```python
from build123d import *

# Parameters (mm, degrees)
SKETCH3_W                                    = 60
SKETCH3_H                                    = 30
BOSS_EXTRUDE1_DEPTH                          = 10
CBORE_FOR_M6_HEX_HEAD_CAP_SCREW1_D           = 6.6
CBORE_FOR_M6_HEX_HEAD_CAP_SCREW1_CBORE_D     = 10.5
CBORE_FOR_M6_HEX_HEAD_CAP_SCREW1_CBORE_DEPTH = 7.5
CUT_EXTRUDE1_DEPTH                           = 10


with BuildPart() as part:
    # Sketch3 → Boss-Extrude1 (new, symmetric)
    with BuildSketch(Plane.XY):
        Rectangle(SKETCH3_W, SKETCH3_H)
    extrude(amount=BOSS_EXTRUDE1_DEPTH, both=True)

    # CBORE for M6 Hex Head Cap Screw1 (through all)
    with Locations(Plane(origin=(0, 0, -10), x_dir=(-1, 0, 0), z_dir=(0, 0, -1))):
        with Locations((18, 0), (-18, 0)):
            CounterBoreHole(CBORE_FOR_M6_HEX_HEAD_CAP_SCREW1_D / 2, CBORE_FOR_M6_HEX_HEAD_CAP_SCREW1_CBORE_D / 2, CBORE_FOR_M6_HEX_HEAD_CAP_SCREW1_CBORE_DEPTH)

    # Sketch9 → Tap Drill for M12 Tap1 (revolve, cut)
    with BuildSketch(Plane(origin=(0, 0, -10), x_dir=(0, 1, 0), z_dir=(1, 0, 0))):
        Polygon((0, 0), (0, 20), (5.125, 20), (5.1, 19.975), (5.1, 0.025), (5.125, 0), align=None)
    revolve(axis=Axis((0, 0, -16.35), (0, 0, 1)), mode=Mode.SUBTRACT)

    # Sketch11 → Cut-Extrude1 (cut)
    with BuildSketch(Plane(origin=(0, 0, 10), x_dir=(-1, 0, 0), z_dir=(0, 0, -1))):
        Polygon((4.907477288, 8.5), (-4.907477288, 8.5), (-9.814954576, 0), (-4.907477288, -8.5), (4.907477288, -8.5), (9.814954576, 0), align=None)
    extrude(amount=CUT_EXTRUDE1_DEPTH, mode=Mode.SUBTRACT)


solid = part.part
```
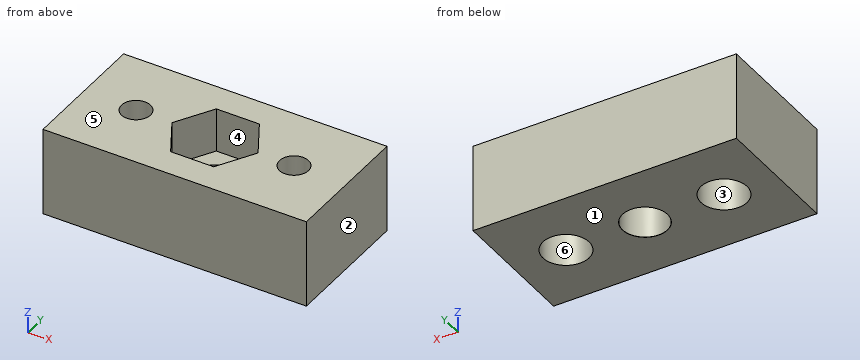
Input: part model. Units: mm. Frame: model coordinates. Face numbers are marked on the shaded views. A direction names the side the tool comes from. Round coordinates to 2 decimals unless told otherwise and drop trailing zeros. Loops run counter-clockwise (first coordinate to the right, second up) from the corner with the lowest first, then second, coordinate; pieces in that order, holes last. Notation, with made-up numbers: (38, 89) -> (51, 89) arc R18 cw to (51, 99) -> close; hole circle Ø9 at (26.5, 0). An arc over 180 degrees is marked (long way). Write each question's results on one line, items separated by ' | '.
1. Mould query, pull axis X, two halves, no side actions, for the marked faces 1, 2 and 3. Classes: +X half, -X half, draft (parallel to the pull), parting line (faces both ways), or undercut.
Geometry results:
face 1: draft | face 2: +X half | face 3: undercut
2. Section D-D (z = -7.75). Return loops of the section in (x, y).
Geometry results:
outline: (-30, -15) -> (30, -15) -> (30, 15) -> (-30, 15) -> close; hole circle Ø10.5 at (-18, 0); hole circle Ø10.2 at (0, 0); hole circle Ø10.5 at (18, 0)
3. First-contact query: P1, Ø8.5, axis at x = 3.5, y = 2.5, coming from the +Z side; P2, Ø5, axis at x = -16.5, y = 1.5, coming from the -Z side. Flat tips, straight axial feed; report the tip coordinate or a pass-through.
Geometry results:
P1: z = 10 | P2: z = -2.5
4. Section B-B (z = 5.5). Return loops of the section in (x, y).
Geometry results:
outline: (-30, -15) -> (30, -15) -> (30, 15) -> (-30, 15) -> close; hole circle Ø6.6 at (-18, 0); hole (-9.81, 0) -> (-4.91, -8.5) -> (4.91, -8.5) -> (9.81, 0) -> (4.91, 8.5) -> (-4.91, 8.5) -> close; hole circle Ø6.6 at (18, 0)
5. Set-up query: the marked faces 4, 5 and 6. Return all of +Z, -Z, +X, -X, +Y, -Y with unobstructed straight access to the full face (end or side cutting, diameter ignored); none if empty.
Geometry results:
face 4: +Z | face 5: +Z, +X, -X, +Y, -Y | face 6: -Z
6. Section C-C (x = 18). Return loops of the section in (y, z), and give its area (3 significant figures).
Geometry results:
outline: (-15, -10) -> (-5.25, -10) -> (-5.25, -2.5) -> (-3.3, -2.5) -> (-3.3, 10) -> (-15, 10) -> close; (3.3, -2.5) -> (5.25, -2.5) -> (5.25, -10) -> (15, -10) -> (15, 10) -> (3.3, 10) -> close | area: 439 mm2
7. Section A-A (x = 0). Return loops of the section in (y, z) (3 decimals).
Geometry results:
outline: (-15, -10) -> (-5.125, -10) -> (-5.1, -9.975) -> (-5.1, 0) -> (-8.5, 0) -> (-8.5, 10) -> (-15, 10) -> close; (5.1, -9.975) -> (5.125, -10) -> (15, -10) -> (15, 10) -> (8.5, 10) -> (8.5, 0) -> (5.1, 0) -> close
8. Ray query, line 1 (Y direction, x = 18, z = -6.75); line 2 (Y direction, x = -18, z = 3.75); line 3 (X direction, y = -0.5, z = -3.5). Return the intervals inside material, ascending. Write a range as from..to.
Geometry results:
line 1: -15..-5.25, 5.25..15 | line 2: -15..-3.3, 3.3..15 | line 3: -30..-23.23, -12.77..-5.08, 5.08..12.77, 23.23..30
